Study the drawing (mm; zero at the part's minimum x, y, z) and answer. Round coordinates to 2 decimals unless told otherwise and drop trailing zeros. Order: outer loops, then holes, each group sorted by start corner. A loop starts at its lowest first (then second) coordinate and runs counter-clockwise, first axis right, second up. Notation, with made-up numbers: (71, 27) - (92, 27) arc R24 cw to (92, 51) - close; hole circle Ø3 at (-8.75, 44.5). An arc over 180 degrees is marked (long way). Put each result on its own line as item: value. Start each with the question number.
Q1. Section B-B on z = 77.15 is taken. Give the vertices of the cut face in (x, y), then the cut area to 3 significant figures.
Q2. This flat-tipped pin is pushed along its axis until it touches: pin 1 Ø3.5 at (x, z) = (6.65, 6.65) entering from +Y (3 decimals). Where does it stop, or does it pass through?
Q3. Find the intervals of material crossed by line 1 along X through (y, z) = (0.9, 147.65); line 2 along Z through (x, y) = (133.65, 1.3); line 3 along X through (y, z) = (1.2, 77.15), in increasing order. Write a range as from..to.
Q4. Section A-A on x = 6.65 is taken. Give the vertices of the cut face in (y, z).
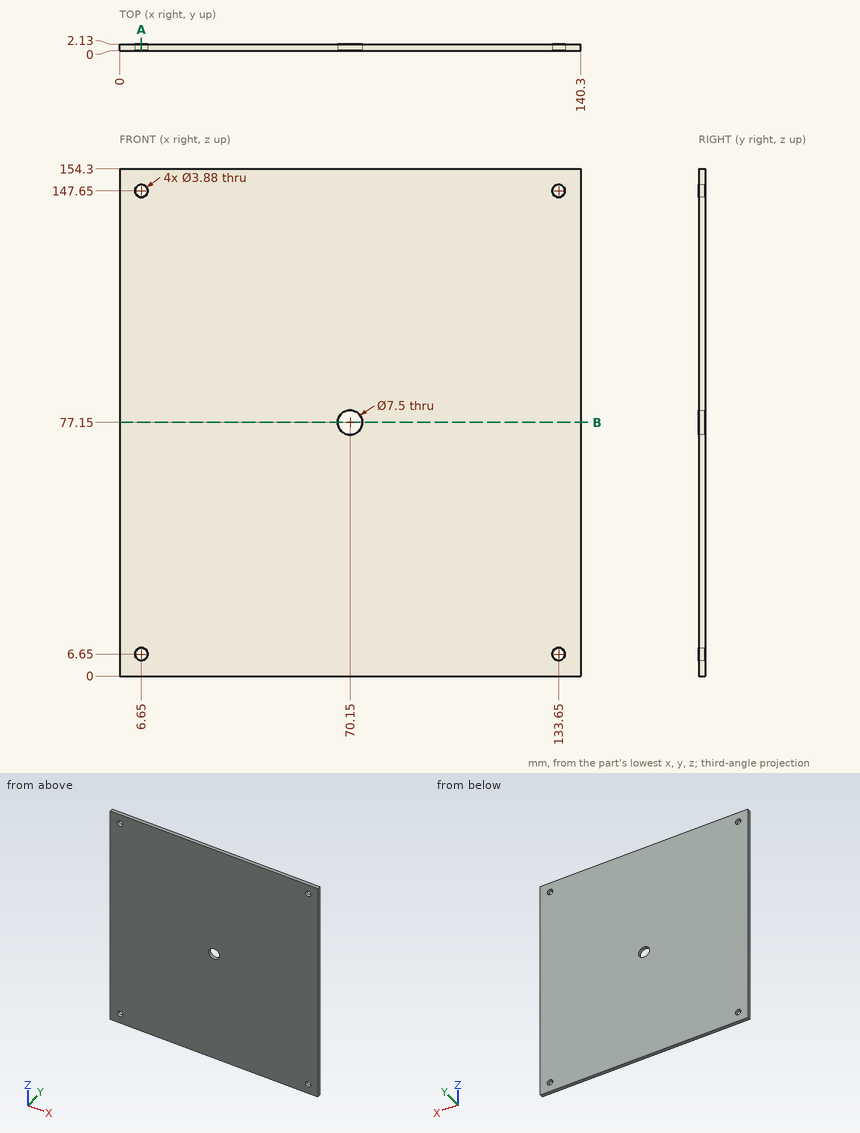
Findings:
1. outline: (0, 0) - (66.4, 0) - (66.4, 2.13) - (0, 2.13) - close; (73.9, 0) - (140.3, 0) - (140.3, 2.13) - (73.9, 2.13) - close
1. area: 283 mm2
2. pin 1: through
3. line 1: 0..4.71, 8.59..131.71, 135.59..140.3
3. line 2: 0..4.71, 8.59..145.71, 149.59..154.3
3. line 3: 0..66.4, 73.9..140.3
4. outline: (0, 0) - (2.13, 0) - (2.13, 4.71) - (0, 4.71) - close; (0, 8.59) - (2.13, 8.59) - (2.13, 145.71) - (0, 145.71) - close; (0, 149.59) - (2.13, 149.59) - (2.13, 154.3) - (0, 154.3) - close
